Can you work these out from the drawing? Everything is in mm from the part's minimum corner. A direction names the side the tool comes from. Round coordinates to 2 decimals unless told otherwise and drop trailing zeros. Order: outer loops, then holes, each group sorted by start corner. A loop starts at its lowest first (then second) coordinate and runs counter-clockwise, first axis right, second up. Notation, with made-up numbers: (80.5, -24.75) - (127.5, -24.75) arc R35 ccw to (127.5, 14.25) - close; hole circle Ø5 at (57.25, 47.25). An arc over 180 degrees is marked (long way). Answer as a JSON object with one key per item and string values.
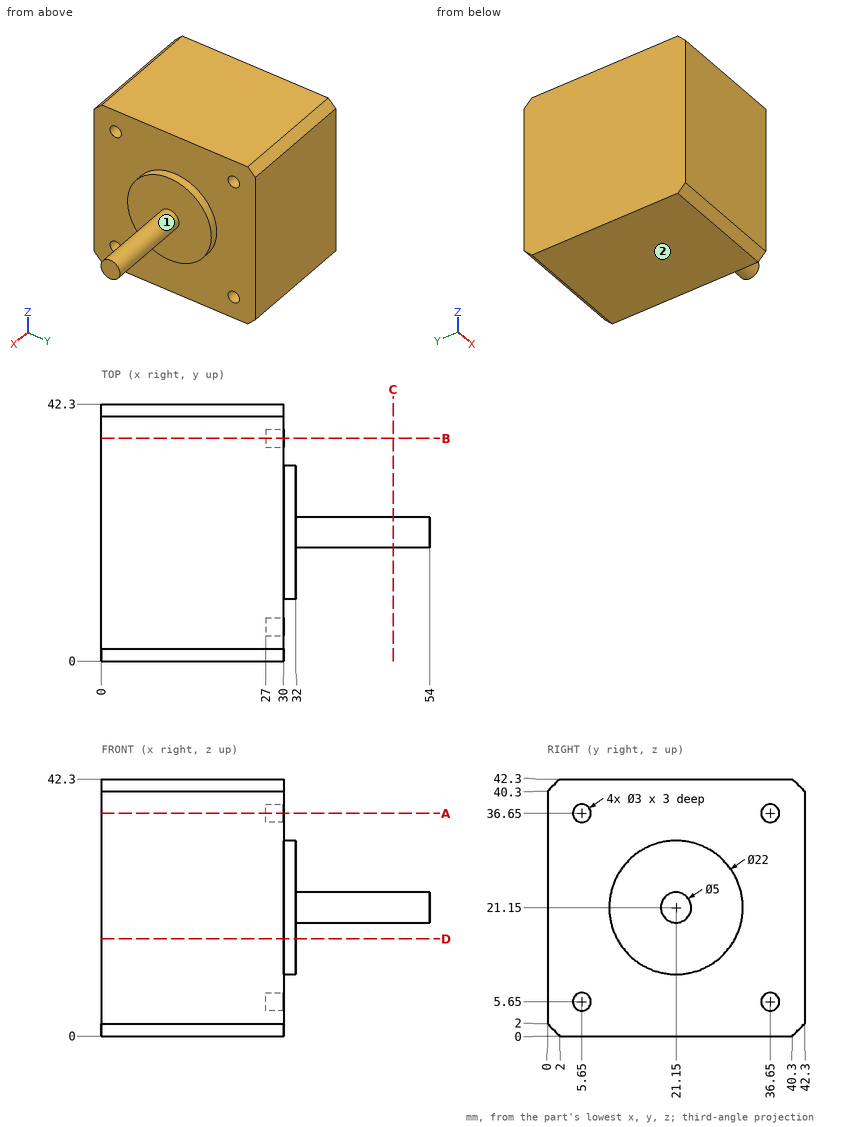
1. Imagine slicing it at C-C (x = 48). List the corners of the cut face in (y, z) for me.
Responses:
{"outline": "circle Ø5 at (21.15, 21.15)"}
2. If I drill on L1, parallel to Y at x = 27.9, z = 5.65; L2, parallel to Y at x = 28, z = 5, over which ranges is the centre line in solid material (lowest first)? Write a range as [from, to].
Responses:
{"L1": "[0, 4.15], [7.15, 35.15], [38.15, 42.3]", "L2": "[0, 4.3], [7, 35.3], [38, 42.3]"}
3. Imagine slicing it at A-A (z = 36.65). List the corners of the cut face in (x, y) for me, plus the area to 3 significant figures.
Responses:
{"outline": "(0, 0) - (30, 0) - (30, 4.15) - (27, 4.15) - (27, 7.15) - (30, 7.15) - (30, 35.15) - (27, 35.15) - (27, 38.15) - (30, 38.15) - (30, 42.3) - (0, 42.3) - close", "area": "1,250 mm2"}
4. Imagine slicing it at D-D (z = 16). List the corners of the cut face in (x, y) for me, plus the area to 3 significant figures.
Responses:
{"outline": "(0, 0) - (30, 0) - (30, 11.43) - (32, 11.43) - (32, 30.87) - (30, 30.87) - (30, 42.3) - (0, 42.3) - close", "area": "1,310 mm2"}
5. For P1, Ø1.8, axis at y = 5.65, z = 36.65, coming from the -X side; P2, Ø3.5, axis at y = 5, z = 5, coming from the +X side; P3, Ø0.9, axis at y = 37, z = 37, coming from the +X side; P4, Ø8, axis at x = 35.5, y = 27.5, coming from the +Z side, each with a flat end and sliding along its axis, tell me the tip position at first contact or that it passes through.
Responses:
{"P1": "x = 0", "P2": "x = 30", "P3": "x = 27", "P4": "z = 31.23"}
6. For the marked faces 1 and 2, which set-ups out of +Z, -Z, +X, -X, +Y, -Y let a thin tool reach every point of the face, with its end or its side?
Responses:
{"face 1": "+X", "face 2": "-Z, +X, -X, +Y, -Y"}
